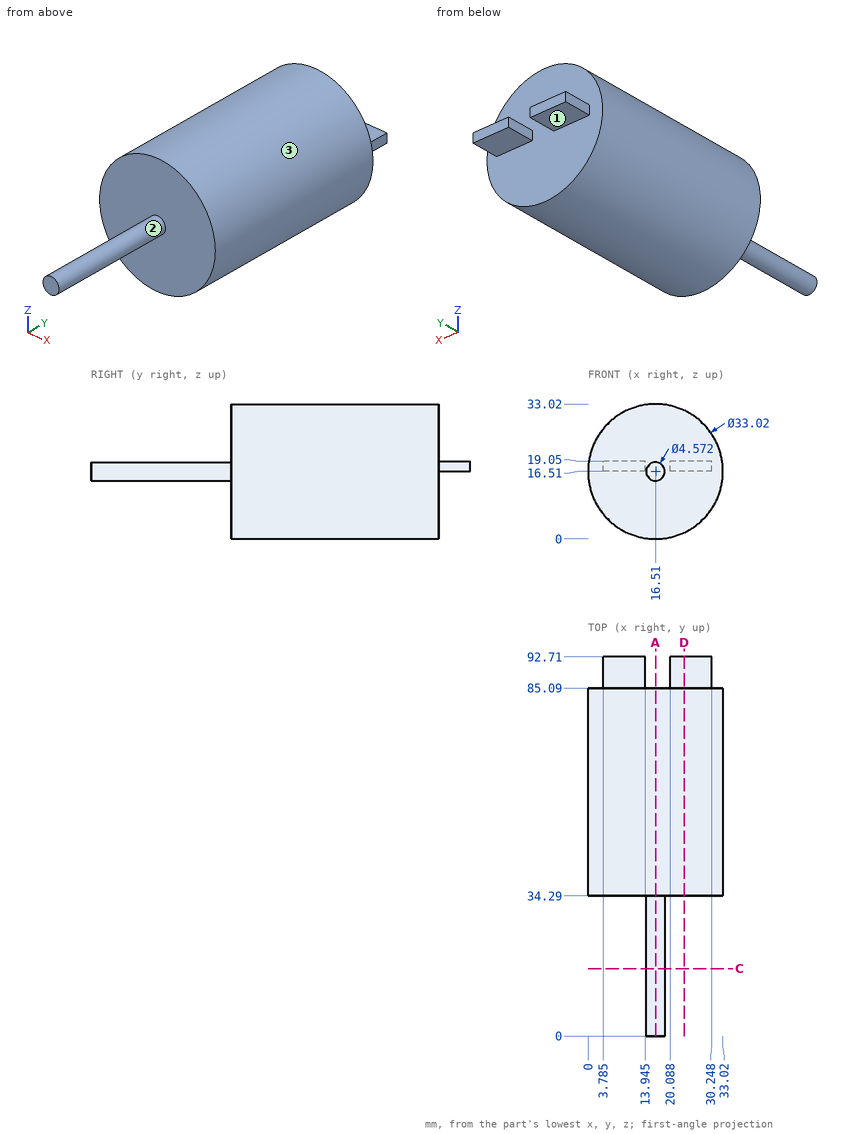
Job drawing, mm, ordinate dimensions from the low corner. One solid piece. A direction names the side the tool comes from. Coordinates: 2 decimals unless noted, no trailing zeros. Write each loop counter-clockwise with the first axis right and the second up, starting at its lowest first coordinate (ties: lowest second). Pieces come first, ordered by that corner, then holes. Notation, with made-up numbers: M 8.25,71 L 43.25,71 A30 ccw 43.25,108 Z; hole C -2.75,57 d1. An arc over 180 degrees is marked long. Answer as a JSON object with one key per item and string values. Group by question number.
1) Wall check: line 1 (Y direction, x = 26, z = 25); line 2 (Z direction, x = 17, y = 42); line 3 (Y direction, x = 26, z = 17.5). Give the ranges that are in metal, low to high. Write a range as from..to.
2) Pin check, flat tips, straight feed: pin 1 Ø10 at (x, y) = (11, 51) entering from -Z; pin 2 Ø2 at (y, z) = (38.5, 25) entering from +X; pin 3 Ø2 at (y, z) = (90.5, 17.5) entering from +X. Stop position of each tip, or through.
3) Saw through at D-D (x = 23.5). Write the cut outline in (y, z).
4) Tool access for the marked faces 1, 2 and 3: list every direction of +Z, -Z, +X, -X, +Y, -Y with a clear straight run to the whole face (end or side of a thin tool).
5) Saw through at C-C (y = 16.5). Write the cut outline in (x, z), plus the area to 3 significant figures.
6) Saw through at A-A (x = 16.51). Write the cut outline in (y, z), plus the area to 3 significant figures.
Values follow:
{
 "1": {"line 1": "y = 34.29..85.09", "line 2": "z = 0.01..33.01", "line 3": "y = 34.29..92.71"},
 "2": {"pin 1": "stops at z = 0.01", "pin 2": "stops at x = 31.22", "pin 3": "stops at x = 30.25"},
 "3": {"outline": "M 34.29,1.55 L 85.09,1.55 L 85.09,16.51 L 92.71,16.51 L 92.71,19.05 L 85.09,19.05 L 85.09,31.47 L 34.29,31.47 Z"},
 "4": {"face 1": "-Z, +X, -X, +Y", "face 2": "-Y", "face 3": "+Y, -Y"},
 "5": {"outline": "C 16.51,16.51 d4.57", "area": "16.4 mm2"},
 "6": {"outline": "M 0,14.22 L 34.29,14.22 L 34.29,0 L 85.09,0 L 85.09,33.02 L 34.29,33.02 L 34.29,18.8 L 0,18.8 Z", "area": "1,830 mm2"}
}
